from build123d import *

# Parameters (mm, degrees)
SKETCH1_W           = 23
SKETCH1_H           = 12
BOSS_EXTRUDE1_DEPTH = 24.1
SKETCH2_R           = 6
SKETCH2_R_2         = 2.7
BOSS_EXTRUDE2_DEPTH = 4.34
BOSS_EXTRUDE4_START = 16.98
SKETCH4_W           = 4.575
SKETCH4_H           = 12
BOSS_EXTRUDE4_DEPTH = 2.42
SKETCH5_R           = 1.5
CUT_EXTRUDE1_DEPTH  = 2.42
FILLET1_R           = 1
FILLET2_R           = 0.5


with BuildPart() as part:
    # Sketch1 → Boss-Extrude1 (new body)
    with BuildSketch(Plane(origin=(0, 0, 0), x_dir=(1, 0, 0), z_dir=(0, 1, 0))):
        Rectangle(SKETCH1_W, SKETCH1_H)
    extrude(amount=BOSS_EXTRUDE1_DEPTH)

    # Sketch2 → Boss-Extrude2 (add)
    with BuildSketch(Plane(origin=(0, 24.1, 0), x_dir=(1, 0, 0), z_dir=(0, 1, 0))):
        with Locations((5.5, 0)):
            Circle(SKETCH2_R)
        Circle(SKETCH2_R_2)
    extrude(amount=BOSS_EXTRUDE2_DEPTH)

    # Sketch4 → Boss-Extrude4 (add)
    with BuildSketch(Plane(origin=(0, 0, 0), x_dir=(1, 0, 0), z_dir=(0, 1, 0)).offset(BOSS_EXTRUDE4_START)):
        with Locations((13.7875, 0)):
            Rectangle(SKETCH4_W, SKETCH4_H)
    boss_extrude4 = extrude(amount=BOSS_EXTRUDE4_DEPTH)

    # Sketch5 → Cut-Extrude1 (cut)
    with BuildSketch(Plane(origin=(0, 19.4, 0), x_dir=(1, 0, 0), z_dir=(0, 1, 0))):
        with Locations((13.65, 0)):
            Circle(SKETCH5_R)
        with BuildLine():
            Line((16.075, 0.7), (14.976649916, 0.7))
            ThreePointArc((14.976649916, 0.7), (15.106017664, 0.360572549), (15.15, 0))
            ThreePointArc((15.15, 0), (15.106017664, -0.360572549), (14.976649916, -0.7))
            Line((14.976649916, -0.7), (16.075, -0.7))
            Line((16.075, -0.7), (16.075, 0.7))
        make_face()
    cut_extrude1 = extrude(amount=-CUT_EXTRUDE1_DEPTH, mode=Mode.SUBTRACT)

    # Mirror2: Boss-Extrude4, Cut-Extrude1 across plane
    add(boss_extrude4.mirror(Plane(origin=(0, 0, 0), x_dir=(0, 0, 1), z_dir=(1, 0, 0))))
    add(cut_extrude1.mirror(Plane(origin=(0, 0, 0), x_dir=(0, 0, 1), z_dir=(1, 0, 0))), mode=Mode.SUBTRACT)

    # Fillet1
    fillet1_edges = [part.edges().sort_by_distance(p)[0] for p in [
        (0.14, 26.27, -2.696367927),
        (0.14, 26.27, 2.696367927),
    ]]
    fillet(fillet1_edges, radius=FILLET1_R)

    # Fillet2
    fillet2_edges = [part.edges().sort_by_distance(p)[0] for p in [
        (11.5, 8.49, 6),
        (11.5, 8.49, -6),
        (16.075, 18.19, -6),
        (16.075, 18.19, 6),
        (-11.5, 8.49, 6),
        (-11.5, 8.49, -6),
        (-16.075, 18.19, -6),
        (-16.075, 18.19, 6),
        (11.5, 21.75, 6),
        (-11.5, 21.75, 6),
        (-11.5, 21.75, -6),
        (11.5, 21.75, -6),
    ]]
    fillet(fillet2_edges, radius=FILLET2_R)


solid = part.part
The model under review builds one solid part; all positions refer to its coordinate system, in mm. A direction names the side the tool comes from. Coordinates: 2 decimals unless noted, no trailing zeros. Write each loop counter-clockwise with the first axis right and the second up, starting at its lowest first coordinate (ties: lowest second). Pieces come first, ordered by that corner, then holes. Notation, with made-up numbers: (48, 81.25) - (68, 81.25) arc R18 cw to (68, 108.25) - close; hole circle Ø4 at (87.25, 58.25). An arc over 180 degrees is marked (long way). Answer as CSV lines item,"result".
(1) We need section D-D (z = 4.75). Give the boundary of the cut face in (x, y) (3 decimals), plus the area to 3 significant figures.
Data:
outline,"(-16.075, 16.98) - (-11.5, 16.98) - (-11.5, 0) - (11.5, 0) - (11.5, 16.98) - (16.075, 16.98) - (16.075, 19.4) - (11.5, 19.4) - (11.5, 24.1) - (9.166, 24.1) - (9.166, 28.44) - (1.834, 28.44) - (1.834, 24.1) - (-11.5, 24.1) - (-11.5, 19.4) - (-16.075, 19.4) - close"
area,"608 mm2"
(2) For line 1 along Z through (x, y) = (-13.65, 18.25); line 2 along Y through (x, z) = (-7, 0.5); line 3 along Y through (x, z) = (13.5, 2), list the stretches that pass through material, from the lowest coordinate up. Write a range as [from, to].
Data:
line 1,"z = [-6, -1.5], [1.5, 6]"
line 2,"y = [0, 24.1]"
line 3,"y = [16.98, 19.4]"
(3) Clearance check with flat-ended pins moving along their axes: pin 1 Ø5.5 at (x, z) = (12.5, 2) entering from -Y; pin 2 Ø5.5 at (x, z) = (-14.5, 1.5) entering from -Y; pin 3 Ø5.5 at (y, z) = (5, 1.5) entering from +X; pin 4 Ø4 at (x, z) = (13.65, 0) entering from +Y. State where each tip first meets the part, or that it passes through.
Data:
pin 1,"stops at y = 0"
pin 2,"stops at y = 16.98"
pin 3,"stops at x = 11.5"
pin 4,"stops at y = 19.4"
(4) We need section A-A (x = 13.65). Give the boundary of the cut face in (y, z), plus the area to 3 significant figures.
Data:
outline,"(16.98, -6) - (19.4, -6) - (19.4, -1.5) - (16.98, -1.5) - close; (16.98, 1.5) - (19.4, 1.5) - (19.4, 6) - (16.98, 6) - close"
area,"21.8 mm2"
(5) Tool access review of faces 1 (the flat face through (-15.5, 18.2, 0.7)), 2 (the cylindrical face through (11.496, 26.24, 0.217)), 3 (the cylindrical face through (-2.7, 26.2, -0.1)), 4 (the flat face through (15.5, 18.2, 0.7)): name each direction out of +Z, -Z, +X, -X, +Y, -Y from which nothing blocks a thin tool from reaching the whole face with its end or side.
Data:
face 1,"-X, +Y, -Y"
face 2,"+Y"
face 3,"-X, +Y"
face 4,"+X, +Y, -Y"
(6) We need section B-B (y = 10). Give the boundary of the cut face in (x, z), plus the area to 3 significant figures.
Data:
outline,"(-11.5, -5.5) arc R0.5 ccw to (-11, -6) - (11, -6) arc R0.5 ccw to (11.5, -5.5) - (11.5, 5.5) arc R0.5 ccw to (11, 6) - (-11, 6) arc R0.5 ccw to (-11.5, 5.5) - close"
area,"276 mm2"
(7) We need section C-C (x = 9). Give the boundary of the cut face in (y, z), plus the area to 3 significant figures.
Data:
outline,"(0, -6) - (24.1, -6) - (24.1, -4.87) - (28.44, -4.87) - (28.44, 4.87) - (24.1, 4.87) - (24.1, 6) - (0, 6) - close"
area,"332 mm2"
